```python
from build123d import *

# Parameters (mm, degrees)
SKETCH1_R           = 0.785
SKETCH1_R_2         = 1.62
BOSS_EXTRUDE1_DEPTH = 7
CUT_EXTRUDE1_DEPTH  = 7


with BuildPart() as part:
    # Sketch1 → Boss-Extrude1 (new body)
    with BuildSketch(Plane(origin=(0, 0, 0), x_dir=(1, 0, 0), z_dir=(0, 1, 0))):
        Polygon((0, 0), (68.005958877, 0), (69.002979439, 0.997020561), (69.002979439, 24.002979439), (68.005958877, 25), (0, 25), (-0.997020561, 24.002979439), (-0.997020561, 0.997020561), align=None)
        with Locations(Location((66.865958877, 2.520750677, 0), (0, 0, 270))):
            Circle(SKETCH1_R, mode=Mode.SUBTRACT)
        with Locations(Location((66.865958877, 22.520750677, 0), (0, 0, 270))):
            Circle(SKETCH1_R, mode=Mode.SUBTRACT)
        with Locations(Location((46.865958877, 22.5, 0), (0, 0, 270))):
            Circle(SKETCH1_R, mode=Mode.SUBTRACT)
        with Locations(Location((46.865958877, 2.5, 0), (0, 0, 270))):
            Circle(SKETCH1_R, mode=Mode.SUBTRACT)
        with Locations(Location((56.865958877, 12.5, 0), (0, 0, 270))):
            Circle(SKETCH1_R_2, mode=Mode.SUBTRACT)
    extrude(amount=BOSS_EXTRUDE1_DEPTH)

    # Sketch2 → Cut-Extrude1 (cut)
    with BuildSketch(Plane(origin=(0, 7, 0), x_dir=(1, 0, 0), z_dir=(0, 1, 0))):
        with BuildLine():
            Line((-0.997020561, 16), (39.002979439, 16))
            ThreePointArc((39.002979439, 16), (42.502979439, 12.5), (39.002979439, 9))
            Line((39.002979439, 9), (-0.997020561, 9))
            ThreePointArc((-0.997020561, 9), (-4.497020561, 12.5), (-0.997020561, 16))
        make_face()
    extrude(amount=-CUT_EXTRUDE1_DEPTH, mode=Mode.SUBTRACT)


solid = part.part
```
Check sheet for the modelled part. Datum: model origin and axes. Units: mm. A direction names the side the tool comes from. Round coordinates to 2 decimals unless told otherwise and drop trailing zeros. Loops run counter-clockwise (first coordinate to the right, second up) from the corner with the lowest first, then second, coordinate; pieces in that order, holes last. Notation, with made-up numbers: (54, 80) -> (74, 80) arc R25 ccw to (74, 115) -> close; hole circle Ø2 at (-31.75, 5.25). An arc over 180 degrees is marked (long way). Answer in a Markdown table with one row per item.
Q1. Sectioned sample at C-C on y = 6. Enter the section's corners in (x, z) (3 decimals), then the cut area to 3 significant figures.
Data:
| item | result |
|---|---|
| outline | (-0.997, -24.003) -> (0, -25) -> (68.006, -25) -> (69.003, -24.003) -> (69.003, -0.997) -> (68.006, 0) -> (0, 0) -> (-0.997, -0.997) -> (-0.997, -9) -> (39.003, -9) arc R3.5 cw to (39.003, -16) -> (-0.997, -16) -> close; hole circle Ø1.57 at (46.866, -22.5); hole circle Ø1.57 at (46.866, -2.5); hole circle Ø3.24 at (56.866, -12.5); hole circle Ø1.57 at (66.866, -22.521); hole circle Ø1.57 at (66.866, -2.521) |
| area | 1,430 mm^2 |
Q2. Set-up check for faces 4 (the face through (19, 4, -9)), 5 (the face through (41.3, 7, -15.5)): record each of +Z, -Z, +X, -X, +Y, -Y from which the full face is reachable in a straight line by a thin tool's end or side.
Data:
| item | result |
|---|---|
| face 4 | -X, +Y, -Y |
| face 5 | +Z, -Z, +X, -X, +Y |
Q3. Go/stop test with flat-tipped pins: P1, Ø1.9, axis at x = 56.87, z = -12.5, coming from the -Y side; P2, Ø1.5, axis at y = 2, z = -11, coming from the -X side. Record where each tip stops, or that it passes through.
Data:
| item | result |
|---|---|
| P1 | passes through |
| P2 | stops at x = 41.68 |
Q4. Release check for a two-part mould opening along Z. For faces 1 (the face through (34, 3, -25)), 2 (the face through (69.003, 3, -12)), 3 (the face through (47.644, 3.451, -2.602)) record: released by +Z, released by -Z, zero draft, split by the parting line, or undercut.
Data:
| item | result |
|---|---|
| face 1 | released by -Z |
| face 2 | zero draft |
| face 3 | undercut |
Q5. Thickness scan on L1, parallel to X at y = 4.5, z = -22.5; L2, parallel to Z at x = 12, y = 4.5; L3, parallel to X at y = 2.75, z = -12.5. Record the ranges inside material, lowest first.
Data:
| item | result |
|---|---|
| L1 | x = -1 to 46.08, 47.65 to 66.08, 67.65 to 69 |
| L2 | z = -25 to -16, -9 to 0 |
| L3 | x = 42.5 to 55.25, 58.49 to 69 |
Q6. Sectioned sample at A-A on z = -12.5. Enter the section's corners in (x, y), then the cut area to 3 significant figures.
Data:
| item | result |
|---|---|
| outline | (42.5, 0) -> (55.25, 0) -> (55.25, 7) -> (42.5, 7) -> close; (58.49, 0) -> (69, 0) -> (69, 7) -> (58.49, 7) -> close |
| area | 163 mm^2 |
Q7. Sectioned sample at B-B on z = -22.5. Enter the section's corners in (x, y).
Data:
| item | result |
|---|---|
| outline | (-1, 0) -> (46.08, 0) -> (46.08, 7) -> (-1, 7) -> close; (47.65, 0) -> (66.08, 0) -> (66.08, 7) -> (47.65, 7) -> close; (67.65, 0) -> (69, 0) -> (69, 7) -> (67.65, 7) -> close |
